Geometry check sheet. Reference: the model listing, model coordinates, mm. A direction names the side the tool comes from. Give positions to 0.01 mm unless a question says otherwise; leave off trailing zeros. Order: outer loops, then holes, each group sorted by start corner. A loop starts at its lowest first (then second) coordinate and runs counter-clockwise, first axis right, second up. Notation, with made-up numbers: M 78.5,63 L 135.5,63 A20 ccw 135.5,71 Z; hole C 14,19 d6. An arc over 180 degrees is marked long. Answer as CSV lines item,"result".
from build123d import *

# Parameters (mm, degrees)
SKETCH1_W           = 35
SKETCH1_H           = 35
BOSS_EXTRUDE1_DEPTH = 30
SKETCH2_R           = 10
BOSS_EXTRUDE2_DEPTH = 15
SKETCH3_R           = 14
BOSS_EXTRUDE3_DEPTH = 7


with BuildPart() as part:
    # Sketch1 → Boss-Extrude1 (new body)
    with BuildSketch(Plane.XY):
        Rectangle(SKETCH1_W, SKETCH1_H)
    extrude(amount=BOSS_EXTRUDE1_DEPTH)

    # Sketch2 → Boss-Extrude2 (add)
    with BuildSketch(Plane.ZY.offset(17.5)):
        with Locations((15, 0)):
            Circle(SKETCH2_R)
    extrude(amount=BOSS_EXTRUDE2_DEPTH)

    # Sketch3 → Boss-Extrude3 (add)
    with BuildSketch(Plane.ZY.offset(32.5)):
        with Locations((15, 0)):
            Circle(SKETCH3_R)
    extrude(amount=BOSS_EXTRUDE3_DEPTH)


solid = part.part
(1) Section check B-B on y = 0. Enter the section's corners in (x, z).
The answers:
outline,"M -39.5,1 L -32.5,1 L -32.5,5 L -17.5,5 L -17.5,0 L 17.5,0 L 17.5,30 L -17.5,30 L -17.5,25 L -32.5,25 L -32.5,29 L -39.5,29 Z"
(2) Material ranges on line 1 (X direction, y = 4, z = 27); line 2 (X direction, y = -13, z = 23); line 3 (Y direction, x = -25, z = 15.5), recorded low to high.
The answers:
line 1,"x = -39.5 to -32.5, -17.5 to 17.5"
line 2,"x = -17.5 to 17.5"
line 3,"y = -9.99 to 9.99"
(3) Section check C-C on z = 26.5. Enter the section's corners in (x, y).
The answers:
outline,"M -39.5,-7.98 L -32.5,-7.98 L -32.5,7.98 L -39.5,7.98 Z; M -17.5,-17.5 L 17.5,-17.5 L 17.5,17.5 L -17.5,17.5 Z"
(4) Tool access check on faces 5 (the face through (-32.5, 3, 5)), 6 (the face through (0, -17.5, 15)), 7 (the face through (-35.951, -5.362, 27.932)). Record the directions out of +Z, -Z, +X, -X, +Y, -Y that give a thin tool (end or side, any length) a straight path to the whole face; none if there is none.
The answers:
face 5,"none"
face 6,"+Z, -Z, +X, -X, -Y"
face 7,"-X"
(5) Section check A-A on z = 15. Enter the section's corners in (x, y), then the cut area to 3 significant figures.
The answers:
outline,"M -39.5,-14 L -32.5,-14 L -32.5,-10 L -17.5,-10 L -17.5,-17.5 L 17.5,-17.5 L 17.5,17.5 L -17.5,17.5 L -17.5,10 L -32.5,10 L -32.5,14 L -39.5,14 Z"
area,"1,720 mm2"
(6) Draft check along X on faces 1 (the face through (0, 17.5, 15)), 2 (the face through (17.5, 0, 15)), 3 (the face through (-24.9, 3, 24.54)), 4 (the face through (-17.5, -0.2, 4.8)). Enter one of: +X half, -X half, draft (parallel to the pull), parting line (faces both ways), or undercut.
The answers:
face 1,"draft"
face 2,"+X half"
face 3,"undercut"
face 4,"undercut"
(7) Section check D-D on x = -18.5. Enter the section's corners in (y, z), then the cut area to 3 significant figures.
The answers:
outline,"C 0,15 d20"
area,"314 mm2"
